```python
from build123d import *

# Parameters (mm, degrees)
SKETCH1_W                                           = 150
SKETCH1_H                                           = 105
BOSS_EXTRUDE1_DEPTH                                 = 5
CBORE_FOR_M4_HEX_SOCKET_HEAD_CAP_SCREW1_D           = 4.5
CBORE_FOR_M4_HEX_SOCKET_HEAD_CAP_SCREW1_CBORE_D     = 8
CBORE_FOR_M4_HEX_SOCKET_HEAD_CAP_SCREW1_CBORE_DEPTH = 4.5
F_5_5_5_5_DIAMETER_HOLE1_D                          = 5.5
SKETCH9_W                                           = 70
SKETCH9_H                                           = 25
CUT_EXTRUDE1_DEPTH                                  = 10
FILLET1_R                                           = 10


with BuildPart() as part:
    # Sketch1 → Boss-Extrude1 (new, symmetric)
    with BuildSketch(Plane(origin=(0, 0, 0), x_dir=(1, 0, 0), z_dir=(0, 1, 0))):
        Rectangle(SKETCH1_W, SKETCH1_H)
    extrude(amount=BOSS_EXTRUDE1_DEPTH, both=True)

    # CBORE for M4 Hex Socket Head Cap Screw1 (through all)
    with Locations(Plane(origin=(0, -5, 0), x_dir=(-1, 0, 0), z_dir=(0, -1, 0))):
        with Locations((-46.5, -25), (-46.5, -10), (-46.5, 10), (-46.5, 25), (46.5, -25), (46.5, -10), (46.5, 10), (46.5, 25)):
            CounterBoreHole(CBORE_FOR_M4_HEX_SOCKET_HEAD_CAP_SCREW1_D / 2, CBORE_FOR_M4_HEX_SOCKET_HEAD_CAP_SCREW1_CBORE_D / 2, CBORE_FOR_M4_HEX_SOCKET_HEAD_CAP_SCREW1_CBORE_DEPTH)

    # Ø5.5 (5.5) Diameter Hole1 (through all)
    with Locations(Plane(origin=(0, 5, 0), x_dir=(1, 0, 0), z_dir=(0, 1, 0))):
        with Locations((65, -42.5), (65, 42.5), (-65, 42.5), (-65, -42.5), (-65, -14), (65, -14), (-65, 14), (65, 14)):
            Hole(F_5_5_5_5_DIAMETER_HOLE1_D / 2)

    # Sketch9 → Cut-Extrude1 (cut)
    with BuildSketch(Plane(origin=(0, 5, 0), x_dir=(1, 0, 0), z_dir=(0, 1, 0))):
        with Locations((0, -40)):
            Rectangle(SKETCH9_W, SKETCH9_H)
    extrude(amount=-CUT_EXTRUDE1_DEPTH, mode=Mode.SUBTRACT)

    # Fillet1
    fillet1_edges = [part.edges().sort_by_distance(p)[0] for p in [
        (-35, 0, 27.5),
        (35, 0, 27.5),
    ]]
    fillet(fillet1_edges, radius=FILLET1_R)


solid = part.part
```
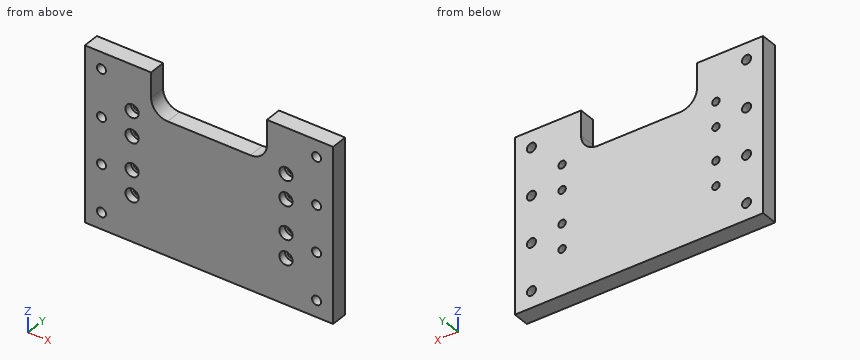
Part model, mm, in its own coordinate system. Round coordinates to 2 decimals unless told otherwise and drop trailing zeros. Loops run counter-clockwise (first coordinate to the right, second up) from the corner with the lowest first, then second, coordinate; pieces in that order, holes last.
Item 1: Cut at C-C, the plane y = -2. State how many separate pieces and enclosed holes the cut face has, then the cut area to 3 significant figures.
Item 2: Cut at B-B, the plane z = -25. Give the cut face in (x, y).
Item 3: Drop a flat-ended pin along its axis: P1, Ø2.5, axis at x = 47.5, z = 12, coming from the -Y side. Give the stop position or say it passes through.
Item 4: Cut at D-D, the plane z = 42.5. Give the cut face in (x, y), then the cut area to 3 significant figures.
Item 5: Cut at A-A, the plane x = 65. Give the cut face in (y, z).
Item 6: Drill centre lines: line 1 (Z direction, x = -65, y = 2.75); line 2 (X direction, y = 3.25, z = -42.5); line 3 (X direction, y = -2.95, z = 25). Where is each one in solid material? Low to high.
A:
1. separate pieces: 1
1. enclosed holes: 16
1. area: 13,500 mm2
2. outline: (-75, -5) - (-50.5, -5) - (-50.5, -0.5) - (-48.75, -0.5) - (-48.75, 5) - (-75, 5) - close; (-44.25, -0.5) - (-42.5, -0.5) - (-42.5, -5) - (42.5, -5) - (42.5, -0.5) - (44.25, -0.5) - (44.25, 5) - (-44.25, 5) - close; (48.75, -0.5) - (50.5, -0.5) - (50.5, -5) - (75, -5) - (75, 5) - (48.75, 5) - close
3. P1: stops at y = -0.5
4. outline: (-75, -5) - (-67.75, -5) - (-67.75, 5) - (-75, 5) - close; (-62.25, -5) - (-35, -5) - (-35, 5) - (-62.25, 5) - close; (35, -5) - (62.25, -5) - (62.25, 5) - (35, 5) - close; (67.75, -5) - (75, -5) - (75, 5) - (67.75, 5) - close
4. area: 690 mm2
5. outline: (-5, -52.5) - (5, -52.5) - (5, -45.25) - (-5, -45.25) - close; (-5, -39.75) - (5, -39.75) - (5, -16.75) - (-5, -16.75) - close; (-5, -11.25) - (5, -11.25) - (5, 11.25) - (-5, 11.25) - close; (-5, 16.75) - (5, 16.75) - (5, 39.75) - (-5, 39.75) - close; (-5, 45.25) - (5, 45.25) - (5, 52.5) - (-5, 52.5) - close
6. line 1: z = -52.5 to -45.25, -39.75 to -16.75, -11.25 to 11.25, 16.75 to 39.75, 45.25 to 52.5
6. line 2: x = -75 to -67.75, -62.25 to 62.25, 67.75 to 75
6. line 3: x = -75 to -50.5, -42.5 to 42.5, 50.5 to 75
